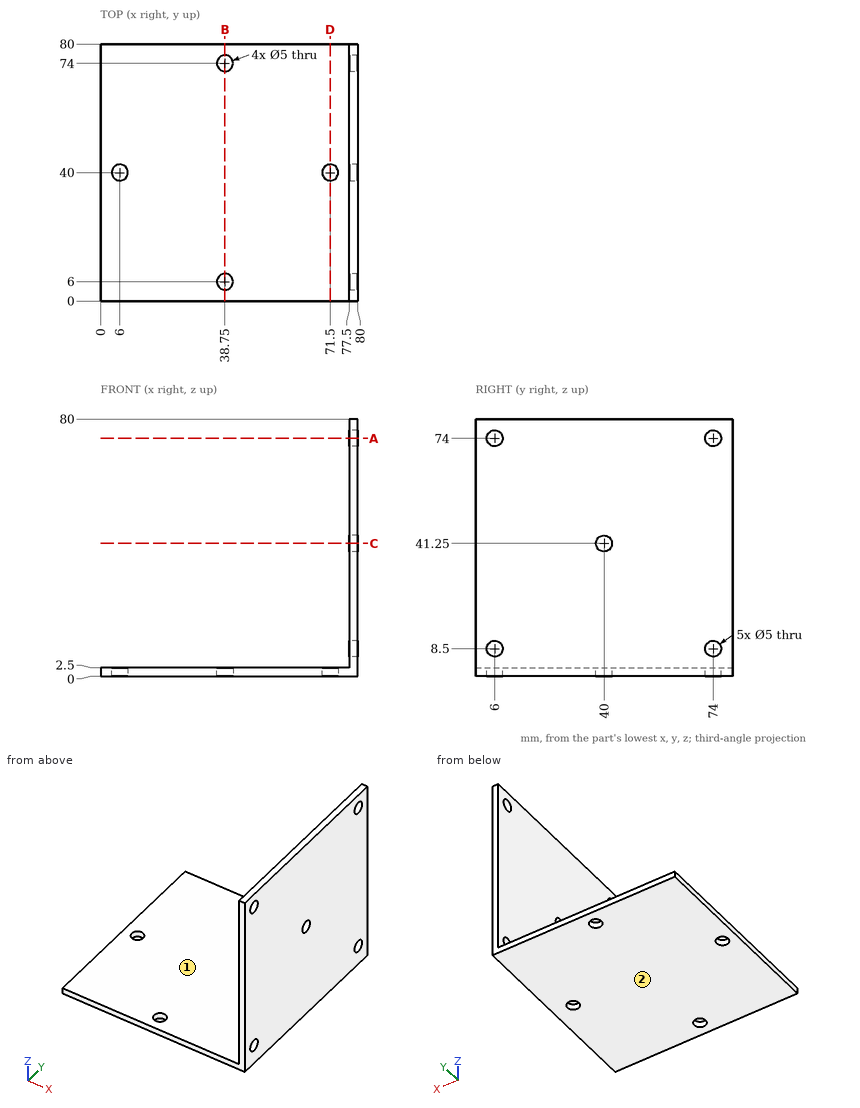
Print and shaded views of the part. All mm, measured from the part's lowest x, y and z. A direction names the side the tool comes from. Round coordinates to 2 decimals unless told otherwise and drop trailing zeros. Write each loop counter-clockwise with the first axis right and the second up, starting at its lowest first coordinate (ties: lowest second). Pieces come first, ordered by that corner, then holes. Notation, with made-up numbers: M 78.5,3.25 L 117.5,3.25 A27 ccw 117.5,32.25 Z; hole C 53,9 d5. An arc over 180 degrees is marked long. Use a Markdown table: item, result. Add a question column.
1. Slice it at B-B on x = 38.75. Give the cut face in (y, z), then the cut area to 3 significant figures.
2. Slice it at A-A on z = 74. Give the cut face in (x, y).
3. Flat gauge pins, fed straight in: P1, Ø3, axis at y = 12.5, z = 49, coming from the -X side; P2, Ø5, axis at x = 42, y = 8, coming from the +Z side. Where does each tip first touch, or does it go through?
4. Slice it at D-D on x = 71.5. Give the cut face in (y, z).
5. Drill centre lines: probe 1 along Z at (x, y) = (79, 74); probe 2 along X at (y, z) = (74, 0.65); probe 3 along Y at (x, z) = (71.5, 1.35). Where is each one in solid material? Low to high.
6. Slice it at C-C on z = 41.25. Give the cut face in (x, y), then the cut area to 4 significant figures.
7. 3-axis set-ups, long thin cutter, end or side, ignore diameter. For the marked faces 1 and 2: which of +Z, -Z, +X, -X, +Y, -Y reach the whole face in a straight line?
Reply:
| question | item | result |
|---|---|---|
| 1 | outline | M 0,0 L 3.5,0 L 3.5,2.5 L 0,2.5 Z; M 8.5,0 L 71.5,0 L 71.5,2.5 L 8.5,2.5 Z; M 76.5,0 L 80,0 L 80,2.5 L 76.5,2.5 Z |
| 1 | area | 175 mm^2 |
| 2 | outline | M 77.5,0 L 80,0 L 80,3.5 L 77.5,3.5 Z; M 77.5,8.5 L 80,8.5 L 80,71.5 L 77.5,71.5 Z; M 77.5,76.5 L 80,76.5 L 80,80 L 77.5,80 Z |
| 3 | P1 | stops at x = 77.5 |
| 3 | P2 | stops at z = 2.5 |
| 4 | outline | M 0,0 L 37.5,0 L 37.5,2.5 L 0,2.5 Z; M 42.5,0 L 80,0 L 80,2.5 L 42.5,2.5 Z |
| 5 | probe 1 | z = 0 to 6, 11 to 71.5, 76.5 to 80 |
| 5 | probe 2 | x = 0 to 36.25, 41.25 to 80 |
| 5 | probe 3 | y = 0 to 37.5, 42.5 to 80 |
| 6 | outline | M 77.5,0 L 80,0 L 80,37.5 L 77.5,37.5 Z; M 77.5,42.5 L 80,42.5 L 80,80 L 77.5,80 Z |
| 6 | area | 187.5 mm^2 |
| 7 | face 1 | +Z, -X, +Y, -Y |
| 7 | face 2 | -Z, +X, -X, +Y, -Y |
